from build123d import *

# Parameters (mm, degrees)
EXTRUDE_1_DEPTH     = 12.5
EXTRUDE_2_DEPTH     = 2.8
SKETCH_3_R          = 5
EXTRUDE_3_DEPTH     = 5
FILLET_1_R          = 5
SKETCH_4_W          = 2.5
SKETCH_4_H          = 3.5
CUT_EXTRUDE_1_DEPTH = 32
SKETCH_5_R          = 3
CUT_EXTRUDE_2_DEPTH = 5


with BuildPart() as part:
    # 草圖1 → 填料-伸長1 (new body, symmetric)
    with BuildSketch(Plane(origin=(0, 0, 0), x_dir=(1, 0, 0), z_dir=(0, 1, 0))):
        with BuildLine():
            Line((-37.5, 5.5), (-15, 5.5))
            Line((-15, 5.5), (-15, 25.5))
            Line((-15, 25.5), (15, 25.5))
            Line((15, 25.5), (15, 5.5))
            Line((15, 5.5), (37.5, 5.5))
            Line((37.5, 5.5), (37.5, -5.5))
            Line((37.5, -5.5), (36, -5.5))
            ThreePointArc((36, -5.5), (30, 0.5), (24, -5.5))
            Line((24, -5.5), (10.392304845, -5.5))
            Line((10.392304845, -5.5), (5.196152423, -14.5))
            Line((5.196152423, -14.5), (-5.196152423, -14.5))
            Line((-5.196152423, -14.5), (-10.392304845, -5.5))
            Line((-10.392304845, -5.5), (-24, -5.5))
            ThreePointArc((-24, -5.5), (-30, 0.5), (-36, -5.5))
            Line((-36, -5.5), (-37.5, -5.5))
            Line((-37.5, -5.5), (-37.5, 5.5))
        make_face()
        Polygon((3.897114317, -12.25), (7.794228634, -5.5), (3.897114317, 1.25), (-3.897114317, 1.25), (-7.794228634, -5.5), (-3.897114317, -12.25), align=None, mode=Mode.SUBTRACT)
    extrude(amount=EXTRUDE_1_DEPTH, both=True)

    # 草圖2 → 填料-伸長2 (add)
    with BuildSketch(Plane(origin=(0, 12.5, 0), x_dir=(1, 0, 0), z_dir=(0, 1, 0))):
        with BuildLine():
            Line((-36, -5.5), (-33.5, -5.5))
            ThreePointArc((-33.5, -5.5), (-30, -2), (-26.5, -5.5))
            Line((-26.5, -5.5), (-24, -5.5))
            ThreePointArc((-24, -5.5), (-30, 0.5), (-36, -5.5))
        make_face()
        with BuildLine():
            Line((26.5, -5.5), (24, -5.5))
            ThreePointArc((24, -5.5), (30, 0.5), (36, -5.5))
            Line((36, -5.5), (33.5, -5.5))
            ThreePointArc((33.5, -5.5), (30, -2), (26.5, -5.5))
        make_face()
    extrude_2 = extrude(amount=-EXTRUDE_2_DEPTH)

    # 鏡射1: 填料-伸長2 across plane
    add(extrude_2.mirror(Plane.ZX))

    # 草圖3 → 填料-伸長3 (add, symmetric)
    with BuildSketch(Plane(origin=(0, 0, 0), x_dir=(1, 0, 0), z_dir=(0, 1, 0))):
        Polygon((7.794228634, -5.5), (3.897114317, 1.25), (-3.897114317, 1.25), (-7.794228634, -5.5), (-3.897114317, -12.25), (3.897114317, -12.25), align=None)
        with Locations((0, -5.5)):
            Circle(SKETCH_3_R, mode=Mode.SUBTRACT)
    extrude(amount=EXTRUDE_3_DEPTH, both=True)

    # 圓角1
    fillet_1_edges = [part.edges().sort_by_distance(p)[0] for p in [
        (-37.5, 0, -5.5),
        (-15, 0, -5.5),
        (-15, 0, -25.5),
        (15, 0, -25.5),
        (15, 0, -5.5),
        (37.5, 0, -5.5),
    ]]
    fillet(fillet_1_edges, radius=FILLET_1_R)

    # 草圖4 → 除料-伸長1 (cut, through all)
    with BuildSketch(Plane.XY.offset(5.5)):
        with Locations((20, 6)):
            Rectangle(SKETCH_4_W, SKETCH_4_H)
        with Locations((20, -6)):
            Rectangle(SKETCH_4_W, SKETCH_4_H)
        with Locations((-20, -6)):
            Rectangle(SKETCH_4_W, SKETCH_4_H)
        with Locations((-20, 6)):
            Rectangle(SKETCH_4_W, SKETCH_4_H)
    extrude(amount=-CUT_EXTRUDE_1_DEPTH, mode=Mode.SUBTRACT)

    # 草圖5 → 除料-伸長2 (cut)
    with BuildSketch(Plane(origin=(0, 12.5, 0), x_dir=(1, 0, 0), z_dir=(0, 1, 0))):
        with Locations((0, 18.5)):
            Circle(SKETCH_5_R)
    extrude(amount=-CUT_EXTRUDE_2_DEPTH, mode=Mode.SUBTRACT)


solid = part.part
Source: CAD feature listing. Evaluate the final solid. Frame: model axes, mm. A direction names the side the tool comes from. Coordinates: 2 decimals unless noted, no trailing zeros. Loops run counter-clockwise (first coordinate to the right, second up) from the corner with the lowest first, then second, coordinate; pieces in that order, holes last. Notation, with made-up numbers: (80, 74) - (118, 74) arc R9 ccw to (118, 81) - close; hole circle Ø2 at (47, -16). An arc over 180 degrees is marked (long way). One line per item, written item: value. Start each with the question number.
1. Ray query, L1, parallel to Z at x = 0, y = 9.1; L2, parallel to Z at x = 0, y = -1.5; L3, parallel to X at y = 8.9, z = -18.5. Return the intervals inside material, ascending.
2. Section D-D (x = -30). Return the cut outline in (y, z), and give its area (3 significant figures).
3. Mould query, pull axis Z, two halves, no side actions, for faces 1 (the cylindrical face through (13.57, -0.18, -24)), 2 (the flat face through (-1, 12.5, -6)), 3 (the flat face through (5.87, 8.8, 2.17)), 4 (the flat face through (-7.76, 0.18, 10.06)). Classes: pulls with the +Z half, pulls with the -Z half, needs draft (parallel to the pull), parting line crosses it, or undercut.
4. Set-up query: faces 5 (the flat face through (-18.75, -6, 0)), 6 (the flat face through (5, 5, 4)), 7 (the flat face through (-15, 0, -15)). Return all of +Z, -Z, +X, -X, +Y, -Y with unobstructed straight access to the full face (end or side cutting, diameter ignored); none if empty.
5. Section A-A (y = -2.5). Return the cut outline in (x, z).
6. Section C-C (z = -18.5). Return the cut outline in (x, y), and give its area (3 significant figures).
7. Contact query for flat-ended pins moving along their axis: P1, Ø3, axis at x = -25.5, y = 7.5, coming from the -Z side; P2, Ø5, axis at y = -3.5, z = -18, coming from the +X side; P3, Ø1, axis at y = 5.5, z = 9.5, coming from the -X side. Output: stop coordinate, or through.
8. Section B-B (x = 0). Return the cut outline in (y, z).
Verdict:
1. L1: z = -25.5 to -21.5, -15.5 to -1.25, 12.25 to 14.5
1. L2: z = -25.5 to 0.5, 10.5 to 14.5
1. L3: x = -15 to -3, 3 to 15
2. outline: (-12.5, -5.5) - (12.5, -5.5) - (12.5, 2) - (9.7, 2) - (9.7, -0.5) - (-9.7, -0.5) - (-9.7, 2) - (-12.5, 2) - close
2. area: 139 mm2
3. face 1: pulls with the -Z half
3. face 2: needs draft
3. face 3: undercut
3. face 4: pulls with the +Z half
4. face 5: +Z, -Z
4. face 6: +Y
4. face 7: -Z, -X, +Y, -Y
5. outline: (-37.5, -0.5) arc R5 ccw to (-32.5, -5.5) - (-20, -5.5) arc R5 cw to (-15, -10.5) - (-15, -20.5) arc R5 ccw to (-10, -25.5) - (10, -25.5) arc R5 ccw to (15, -20.5) - (15, -10.5) arc R5 cw to (20, -5.5) - (32.5, -5.5) arc R5 ccw to (37.5, -0.5) - (37.5, 5.5) - (36, 5.5) arc R6 cw to (24, 5.5) - (10.39, 5.5) - (5.2, 14.5) - (-5.2, 14.5) - (-10.39, 5.5) - (-24, 5.5) arc R6 cw to (-36, 5.5) - (-37.5, 5.5) - close; hole circle Ø10 at (0, 5.5)
6. outline: (-15, -12.5) - (15, -12.5) - (15, 12.5) - (3, 12.5) - (3, 7.5) - (-3, 7.5) - (-3, 12.5) - (-15, 12.5) - close
6. area: 720 mm2
7. P1: stops at z = -5.5
7. P2: stops at x = 15
7. P3: stops at x = -8.37
8. outline: (-12.5, -25.5) - (12.5, -25.5) - (12.5, -21.5) - (7.5, -21.5) - (7.5, -15.5) - (12.5, -15.5) - (12.5, -1.25) - (5, -1.25) - (5, 0.5) - (-5, 0.5) - (-5, -1.25) - (-12.5, -1.25) - close; (-12.5, 12.25) - (-5, 12.25) - (-5, 10.5) - (5, 10.5) - (5, 12.25) - (12.5, 12.25) - (12.5, 14.5) - (-12.5, 14.5) - close
